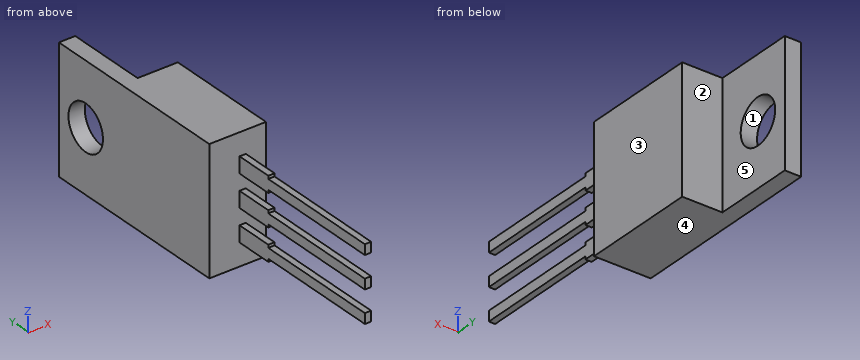
Autodesk Inventor part; units mm, degrees
ref_plane "YZ Plane" through (0, 0, 0) normal (1, 0, 0) x (0, 1, 0)
ref_plane "XZ Plane" through (0, 0, 0) normal (0, 1, 0) x (-1, 0, 0)
ref_plane "XY Plane" through (0, 0, 0) normal (0, 0, 1) x (1, 0, 0)
sketch "Boceto1" plane through (0, 0, 0) normal (0, 1, 0) x (-1, 0, 0)
  line L0 (2.25, 4.95) -> (-2.25, 4.95)
  line L1 (-2.25, 4.95) -> (-2.25, -4.95)
  line L2 (-2.25, -4.95) -> (2.25, -4.95)
  line L3 (2.25, -4.95) -> (2.25, 4.95)
  point P0 (0, 0)
  dimension "d0" = 4.5
  dimension "d1" = 9.9
  dimension "d2" = 4.95
  dimension "d3" = 2.25
extrude "Extrusión1" add sketch "Boceto1" along normal mid plane 9.2
sketch "Boceto2" plane through (0, 4.6, 0) normal (0, 1, 0) x (1, 0, 0)
  line L0 (2.25, 4.95) -> (-2.25, 4.95)
  line L1 (-2.25, 4.95) -> (-2.25, -4.95)
  line L2 (-2.25, -4.95) -> (2.25, -4.95)
  line L3 (2.25, -4.95) -> (2.25, 4.95)
  line L4 (2.25, 4.95) -> (-2.25, 4.95)
  line L5 (-2.25, -4.95) -> (-0.95, -4.95)
  line L6 (-0.95, -4.95) -> (-0.95, 4.95)
  line L7 (-0.95, 4.95) -> (-2.25, 4.95)
  line L8 (-2.25, 4.95) -> (-2.25, -4.95)
  point P0 (0, 0)
  point P1 (-0.95, 4.95)
  dimension "d6" = 1.3
extrude "Extrusión2" add sketch "Boceto2" along normal blind 6.5 contours L6 L2 L1 L0
sketch "Boceto3" plane through (-0.95, 4.6, 4.95) normal (1, 0, 0) x (0, 0, -1)
  line L0 (9.9, 0) -> (0, 0)
  line L1 (9.9, 0) -> (9.9, 6.5)
  line L2 (0, 6.5) -> (9.9, 6.5)
  line L3 (0, 0) -> (0, 6.5)
  circle A0 centre (4.95, 3.7) radius 1.8
  point P0 (4.95, -4.6)
  dimension "d9" = 3.6
  dimension "d10" = 4.95
  dimension "d11" = 3.7
extrude "Extrusión3" cut sketch "Boceto3" against normal blind 6.5 contours A0
sketch "Boceto4" plane through (0, -4.6, 0) normal (0, -1, 0) x (1, 0, 0)
  line L0 (-2.25, -4.95) -> (2.25, -4.95)
  line L1 (2.25, -4.95) -> (2.25, 4.95)
  line L2 (2.25, 4.95) -> (-2.25, 4.95)
  line L3 (-2.25, 4.95) -> (-2.25, -4.95)
  line L4 (0.65, 3.175) -> (0.15, 3.175)
  line L5 (0.15, 3.175) -> (0.15, 1.905)
  line L6 (0.15, 1.905) -> (0.65, 1.905)
  line L7 (0.65, 1.905) -> (0.65, 3.175)
  line L8 (0.65, 0.635) -> (0.15, 0.635)
  line L9 (0.15, 0.635) -> (0.15, -0.635)
  line L10 (0.15, -0.635) -> (0.65, -0.635)
  line L11 (0.65, -0.635) -> (0.65, 0.635)
  line L12 (0.65, -1.905) -> (0.15, -1.905)
  line L13 (0.15, -1.905) -> (0.15, -3.175)
  line L14 (0.15, -3.175) -> (0.65, -3.175)
  line L15 (0.65, -3.175) -> (0.65, -1.905)
  point P0 (0, 0)
  dimension "d14" = 1.27
  dimension "d15" = 1.27
  dimension "d16" = 1.27
  dimension "d17" = 0.5
  dimension "d18" = 0.5
  dimension "d19" = 0.5
  dimension "d20" = 1.27
  dimension "d21" = 1.27
  dimension "d22" = 4.315
  dimension "d23" = 2.4
extrude "Extrusión4" add sketch "Boceto4" along normal blind 3 contours L7 L6 L5 L4 | L11 L10 L9 L8 | L15 L14 L13 L12
sketch "Boceto5" plane through (0, -7.6, 0) normal (0, -1, 0) x (1, 0, 0)
  line L0 (0.15, 3.175) -> (0.15, 1.905)
  line L1 (0.15, 1.905) -> (0.65, 1.905)
  line L2 (0.65, 1.905) -> (0.65, 3.175)
  line L3 (0.65, 3.175) -> (0.15, 3.175)
  line L4 (0.15, 0.635) -> (0.15, -0.635)
  line L5 (0.15, -0.635) -> (0.65, -0.635)
  line L6 (0.65, -0.635) -> (0.65, 0.635)
  line L7 (0.65, 0.635) -> (0.15, 0.635)
  line L8 (0.65, -1.905) -> (0.15, -1.905)
  line L9 (0.15, -1.905) -> (0.15, -3.175)
  line L10 (0.15, -3.175) -> (0.65, -3.175)
  line L11 (0.65, -3.175) -> (0.65, -1.905)
  line L12 (0.15, 1.905) -> (0.15, 3.175)
  line L13 (0.65, 2.94) -> (0.15, 2.94)
  line L14 (0.15, 2.94) -> (0.15, 2.14)
  line L15 (0.15, 2.14) -> (0.65, 2.14)
  line L16 (0.65, 2.14) -> (0.65, 2.94)
  line L17 (0.15, 0.635) -> (0.15, -0.635)
  line L18 (0.65, 0.4) -> (0.15, 0.4)
  line L19 (0.15, 0.4) -> (0.15, -0.4)
  line L20 (0.15, -0.4) -> (0.65, -0.4)
  line L21 (0.65, -0.4) -> (0.65, 0.4)
  line L22 (0.65, -1.905) -> (0.65, -3.175)
  line L23 (0.15, -3.175) -> (0.15, -1.905)
  line L24 (0.65, -2.14) -> (0.15, -2.14)
  line L25 (0.15, -2.14) -> (0.15, -2.94)
  line L26 (0.15, -2.94) -> (0.65, -2.94)
  line L27 (0.65, -2.94) -> (0.65, -2.14)
  point P0 (0, 0)
  point P1 (0.15, -2.14)
  dimension "d26" = 0.8
  dimension "d27" = 0.8
  dimension "d28" = 0.8
  dimension "d29" = 0.235
  dimension "d30" = 0.235
  dimension "d31" = 0.235
extrude "Extrusión5" add sketch "Boceto5" along normal blind 10.08 contours L13 L2 L15 L0 | L18 L6 L20 L4 | L11 L26 L9 L24
sketch "Boceto6" plane through (2.25, -4.6, -4.95) normal (1, 0, 0) x (0, 0, -1)
  line L0 (-8.7824, 7.8194) -> (-0.868, 7.8194) construction
  line L1 (-0.868, 7.8194) -> (-0.868, 3.7441) construction
  line L2 (-0.868, 3.7441) -> (-8.7824, 3.7441) construction
  line L3 (-8.7824, 3.7441) -> (-8.7824, 7.8194) construction
  point P0 (-4.95, 4.6)
properties part number "7805"
Verification items for the finished model (mm, model axes). Face numbers are marked on the shaded views. A direction names the side the tool comes from. Coordinates: 2 decimals unless noted, no trailing zeros. Write each loop counter-clockwise with the first axis right and the second up, starting at its lowest first coordinate (ties: lowest second). Pieces come first, ordered by that corner, then holes. Notation, with made-up numbers: M 61,29.25 L 88,29.25 A17 cw 88,47.25 Z; hole C 6,-3 d8. An arc over 180 degrees is marked long. One line per question, with ' | ' between items.
1) Sectioned sample at A-A on y = 8.3. Record the cut outline in (x, z), then the cut area to 3 significant figures.
Solutions:
outline: M -2.25,-4.95 L -0.95,-4.95 L -0.95,-1.8 L -2.25,-1.8 Z; M -2.25,1.8 L -0.95,1.8 L -0.95,4.95 L -2.25,4.95 Z | area: 8.19 mm^2
2) Sectioned sample at D-D on z = -2.5. Record the cut outline in (x, y), then the cut area to 3 significant figures.
Solutions:
outline: M -2.25,-4.6 L 0.15,-4.6 L 0.15,-17.68 L 0.65,-17.68 L 0.65,-4.6 L 2.25,-4.6 L 2.25,4.6 L -0.95,4.6 L -0.95,11.1 L -2.25,11.1 Z | area: 56.4 mm^2
3) Access from +Z, -Z, +X, -X, +Y, -Y to the whole of each face (thin tool, end or side, straight path). Record for the marked faces 4 and 5.
Solutions:
face 4: -Z, +X, -X, +Y, -Y | face 5: +Z, -Z, +X, +Y
4) Material ranges on L1, parallel to Z at x = 0.25, y = -12.25; L2, parallel to Y at x = -1.45, z = 0; L3, parallel to Y at x = 1.45, z = 0.5, recorded low to high.
Solutions:
L1: -2.94 to -2.14, -0.4 to 0.4, 2.14 to 2.94 | L2: -4.6 to 6.5, 10.1 to 11.1 | L3: -4.6 to 4.6
5) Sectioned sample at B-B on z = 0. Record the cut outline in (x, y), then the cut area to 3 significant figures.
Solutions:
outline: M -2.25,-4.6 L 0.15,-4.6 L 0.15,-17.68 L 0.65,-17.68 L 0.65,-4.6 L 2.25,-4.6 L 2.25,4.6 L -0.95,4.6 L -0.95,6.5 L -2.25,6.5 Z; M -2.25,10.1 L -0.95,10.1 L -0.95,11.1 L -2.25,11.1 Z | area: 51.7 mm^2
6) Sectioned sample at C-C on y = -6.5. Record the cut outline in (x, z) (3 decimals).
Solutions:
outline: M 0.15,-3.175 L 0.65,-3.175 L 0.65,-1.905 L 0.15,-1.905 Z; M 0.15,-0.635 L 0.65,-0.635 L 0.65,0.635 L 0.15,0.635 Z; M 0.15,1.905 L 0.65,1.905 L 0.65,3.175 L 0.15,3.175 Z
7) Depth check by flat-ended pin: pin 1 Ø3 at (y, z) = (8.3, 0) entering from -X; pin 2 Ø0.6 at (x, y) = (0.5, -7) entering from -Z (3 decimals); pin 3 Ø4 at (y, z) = (-13.5, -1.5) entering from +X; pin 4 Ø0.6 at (x, y) = (0.5, -11) entering from -Z. Enter the tip coordinate at first touch or a pass-through.
Solutions:
pin 1: through | pin 2: z = -3.175 | pin 3: x = 0.65 | pin 4: z = -2.94
8) Release check for a two-part mould opening along Y. For the marked faces 1, 2 and 3 record: +Y half, -Y half, draft (parallel to the pull), parting line (faces both ways), or undercut.
Solutions:
face 1: undercut | face 2: +Y half | face 3: draft
